For this review, take the finished solid that the model builds, in its own axes (mm). A direction names the side the tool comes from. Round coordinates to 2 decimals unless told otherwise and drop trailing zeros. Loops run counter-clockwise (first coordinate to the right, second up) from the corner with the lowest first, then second, coordinate; pieces in that order, holes last. Notation, with made-up numbers: M 76,86 L 81,86 A24 ccw 81,123 Z; hole C 38,33.5 d11. An arc over 180 degrees is marked long. One line per question, with ' | ' between items. Start each with the question number.
1) We need section C-C (x = 5). Give the boundary of the cut face in (y, z), and give its area (3 significant figures).
2) Mouldability with a two-part tool opening along X and no side actions: class faces 5 (the face through (-0.21, -31.76, -3.71)), 6 (the face through (0, 0, 3)) as pulls with the +X half, pulls with the -X half, needs draft (parallel to the pull), parting line crosses it, or undercut.
3) For pin 1 Ø1.6 at (x, z) = (-2, 3.5) entering from +Y; pin 2 Ø20 at (x, y) = (-22.5, 13) entering from -Z; pin 3 Ø2.5 at (x, z) = (-11, 3) entering from +Y; pin 4 Ø3.5 at (y, z) = (-33.5, -1.5) entering from -X, all flat-tipped, find the tip position at first contact; note any pin that passes through.
4) We need section D-D (y = 29.5). Give the boundary of the cut face in (x, z), and give its area (4 significant figures).
5) For faces 1 (the face through (32.6, 0.2, 0)), 2 (the face through (-32, 0, 0)), 3 (the face through (-31.25, 0, 1)), 4 (the face through (0, -18.5, 4)), list the 3-axis set-ups (+Z, -Z, +X, -X, +Y, -Y) from which the entire face can be reached by the end or side of a thin tool; tool diameter is ignored.
6) We need section A-A (z = -1.05). Give the boundary of the cut face in (x, y), and give its area (3 significant figures).
7) For probe 1 along X at (y, z) = (-1, 1); probe 2 along Z at (x, y) = (-26.5, -4.5), list the stretches that pass through material, from the lowest coordinate up. Write a range as from..to.
8) We need section B-B (y = -23.5). Give the boundary of the cut face in (x, z), and give its area (3 significant figures).
```python
from build123d import *

# Parameters (mm, degrees)
SKETCH_W        = 66
SKETCH_H        = 66
PAD_DEPTH       = 5
SKETCH001_W     = 62.5
SKETCH001_H     = 62.5
POCKET_DEPTH    = 3
POCKET001_DEPTH = 2
PAD001_DEPTH    = 15
FILLET_R        = 1
FILLET001_R     = 1
FILLET002_R     = 8
FILLET003_R     = 8


with BuildPart() as part:
    # Sketch → Pad (new body)
    with BuildSketch(Plane.XY):
        Rectangle(SKETCH_W, SKETCH_H)
    extrude(amount=PAD_DEPTH)

    # Sketch001 (on Face5 of Pad) → Pocket (cut)
    with BuildSketch(Plane(origin=(0, 0, 0), x_dir=(1, 0, 0), z_dir=(0, 0, -1))):
        Rectangle(SKETCH001_W, SKETCH001_H)
    extrude(amount=-POCKET_DEPTH, mode=Mode.SUBTRACT)

    # Sketch002 (on Face5 of Pocket) → Pocket001 (cut)
    with BuildSketch(Plane.XY.offset(5)):
        with BuildLine():
            ThreePointArc((-6.5, -18.5), (-11.5, -23.5), (-6.5, -28.5))
            Line((-6.5, -28.5), (6.5, -28.5))
            ThreePointArc((6.5, -28.5), (11.5, -23.5), (6.5, -18.5))
            Line((6.5, -18.5), (-6.5, -18.5))
        make_face()
    extrude(amount=-POCKET001_DEPTH, mode=Mode.SUBTRACT)

    # Sketch003 (on DatumPlane) → Pad001 (join, symmetric)
    with BuildSketch(Plane(origin=(0, -33, 5), x_dir=(0, 1, 0), z_dir=(1, 0, 0))):
        with BuildLine():
            ThreePointArc((1.75, -5), (0.7, -6.05), (1.75, -7.1))
            Line((1.75, -7.1), (1.75, -9.1))
            ThreePointArc((1.75, -3), (-1.3, -6.05), (1.75, -9.1))
            Line((1.75, -5), (1.75, -3))
        make_face()
        with BuildLine():
            ThreePointArc((64.25, -7.1), (65.3, -6.05), (64.25, -5))
            Line((64.25, -5), (64.25, -3))
            ThreePointArc((64.25, -9.1), (67.3, -6.05), (64.25, -3))
            Line((64.25, -7.1), (64.25, -9.1))
        make_face()
    extrude(amount=PAD001_DEPTH, both=True)

    # Fillet
    fillet_edges = [part.edges().sort_by_distance(p)[0] for p in [
        (0, 31.25, -4.1),
    ]]
    fillet(fillet_edges, radius=FILLET_R)

    # Fillet001
    fillet001_edges = [part.edges().sort_by_distance(p)[0] for p in [
        (0, -31.25, -4.1),
    ]]
    fillet(fillet001_edges, radius=FILLET001_R)

    # Fillet002
    fillet002_edges = [part.edges().sort_by_distance(p)[0] for p in [
        (0, -33, 1.447999),
    ]]
    fillet(fillet002_edges, radius=FILLET002_R)

    # Fillet003
    fillet003_edges = [part.edges().sort_by_distance(p)[0] for p in [
        (0, 33, 1.447999),
    ]]
    fillet(fillet003_edges, radius=FILLET003_R)


solid = part.part
```
Answers below:
1) outline: M -33.94,0.39 A3.05 ccw -32.74,-3.71 A1 ccw -31.25,-2.84 L -31.25,-2.1 A1.05 cw -31.25,0 L -31.25,3 L -28.5,3 L -28.5,5 L -33,5 L -33,4.15 A8 cw Z; M -18.5,3 L 31.25,3 L 31.25,0 A1.05 cw 31.25,-2.1 L 31.25,-2.84 A1 ccw 32.74,-3.71 A3.05 ccw 33.94,0.39 A8 cw 33,4.15 L 33,5 L -18.5,5 Z | area: 142 mm^2
2) face 5: needs draft | face 6: undercut
3) pin 1: y = 33.13 | pin 2: z = 0 | pin 3: y = 33.37 | pin 4: x = -33
4) outline: M -33,0 L -31.25,0 L -31.25,3 L 31.25,3 L 31.25,0 L 33,0 L 33,5 L -33,5 Z | area: 142.5 mm^2
5) face 1: -Z, +X, +Y, -Y | face 2: -Z, -X, +Y, -Y | face 3: -Z | face 4: +Z, -Z
6) outline: M -15,-34.3 L 15,-34.3 L 15,-32.3 L -15,-32.3 Z; M -15,32.3 L 15,32.3 L 15,34.3 L -15,34.3 Z | area: 120 mm^2
7) probe 1: -33..-31.25, 31.25..33 | probe 2: 3..5
8) outline: M -33,0 L -31.25,0 L -31.25,3 L -11.5,3 L -11.5,5 L -33,5 Z; M 11.5,3 L 31.25,3 L 31.25,0 L 33,0 L 33,5 L 11.5,5 Z | area: 96.5 mm^2
